Source: CAD feature listing. Evaluate the final solid. Frame: model axes, mm. Face numbers are marked on the shaded views. A direction names the side the tool comes from. Give positions to 0.01 mm unless a question says otherwise; leave off trailing zeros. Write each loop counter-clockwise with the first axis right and the second up, starting at its lowest first coordinate (ties: lowest second). Pieces come first, ordered by that corner, then holes. Notation, with made-up numbers: M 51,17.5 L 82,17.5 A20 cw 82,34.5 Z; hole C 51,75 d6. An arc over 180 degrees is marked long. Return JSON: item names as keys, results as strings.
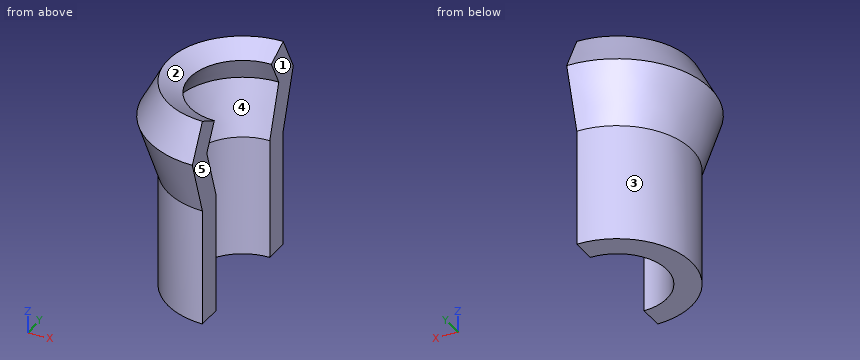
```python
from build123d import *

# Parameters (mm, degrees)
F1_ANGLE = 180


with BuildPart() as f1:
    # F0 (on Front) → F1 (revolve, symmetric)
    with BuildSketch(Plane.XZ) as f1_sk:
        Polygon((-30.562608, 38.93813), (-33.217363, 40.335368), (-35.477046, 36.041968), (-33.217363, 29.036945), (-33.217363, 14.800933), (-30.217363, 14.800933), (-30.217363, 29.508843), (-32.234412, 35.7617), align=None)
    revolve(axis=Axis((-24.178624, 0, 27.116214), (0, 0, -1)), revolution_arc=F1_ANGLE / 2)
    revolve(f1_sk.sketch, axis=Axis((-24.178624, 0, 27.116214), (0, 0, 1)), revolution_arc=F1_ANGLE / 2)


solid = f1.part
```
1) Draft query along Y for the marked faces 1, 2 and 3. Return one class per face: released by +Y, released by -Y, zero draft, split by the parting line, or undercut.
Numbers:
{"face 1": "zero draft", "face 2": "undercut", "face 3": "split by the parting line"}
2) Set-up query: the marked faces 4 and 5. Return all of +Z, -Z, +X, -X, +Y, -Y with unobstructed straight access to the full face (end or side cutting, diameter ignored); none if empty.
Numbers:
{"face 4": "+X", "face 5": "+Z, -Z, +X, +Y, -Y"}
3) Contact query for flat-ended pins moving along their axis: pin 1 Ø1.5 at (y, z) = (-1.5, 27) entering from +X; pin 2 Ø4 at (y, z) = (6, 28) entering from +X; pin 3 Ø6 at (x, z) = (-32.5, 21) entering from +Y; pin 4 Ø1.5 at (x, z) = (-27, 28) entering from -Y. Output: stop coordinate, or through.
Numbers:
{"pin 1": "stops at x = -29.78", "pin 2": "stops at x = -24.18", "pin 3": "stops at y = 7.31", "pin 4": "stops at y = -8.8"}
4) Cut plane A-A, the plane y = 0. Return the cut outline in (x, z).
Numbers:
{"outline": "M -35.48,36.04 L -33.22,29.04 L -33.22,14.8 L -30.22,14.8 L -30.22,29.51 L -32.23,35.76 L -30.56,38.94 L -33.22,40.34 Z"}
5) Cut plane B-B, the plane z = 21.5. Return the cut outline in (x, y), then the cut area to 3 significant figures.
Numbers:
{"outline": "M -24.18,-9.04 L -24.18,-6.04 A6.04 cw -24.18,6.04 L -24.18,9.04 A9.04 ccw Z", "area": "71.1 mm²"}
6) Line query: line 1 (Y direction, x = -27.5, z = 30.5); line 2 (Z direction, x = -30, y = -4.75); line 3 (Y direction, x = -27, z = 38.75). Output: solid intervals per line, ascending. Write a range as [from, to].
Numbers:
{"line 1": "y = [-8.91, -5.42], [5.42, 8.91]", "line 2": "z = [14.8, 34.08], [36.79, 39.53]", "line 3": "y = [-9.46, -5.84], [5.84, 9.46]"}
